```python
from build123d import *

# Parameters (mm, degrees)
F0_W     = 15
F0_H     = 22.5
F1_DEPTH = 0.75
F2_DEPTH = 2


with BuildPart() as f1:
    # F0 (on Top) → F1 (new body)
    with BuildSketch(Plane.XY):
        with Locations((-24.588022, -15.75)):
            Rectangle(F0_W, F0_H)
        Polygon((-18.888022, -25), (-30.888022, -25), (-30.888022, -10), (-21.388022, -10), (-18.888022, -12.5), align=None, mode=Mode.SUBTRACT)
    extrude(amount=F1_DEPTH)

    # F0 (on Top) → F2 (join)
    with BuildSketch(Plane.XY):
        Polygon((-32.088022, 3), (-32.088022, -4.5), (-17.088022, -4.5), (-17.088022, 0), (-20.088022, 3), align=None)
    extrude(amount=F2_DEPTH)


solid = f1.part
```
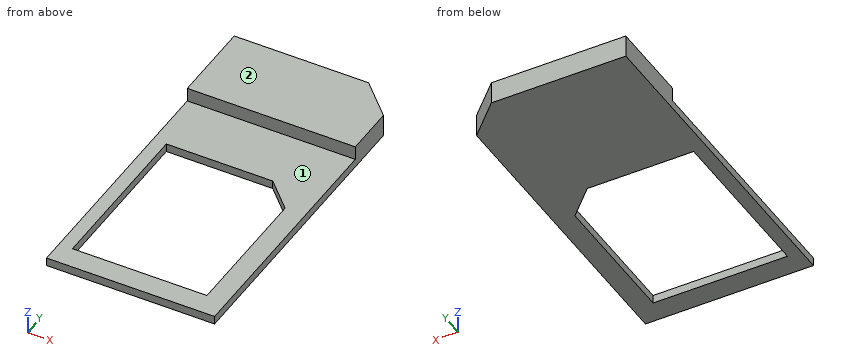
The listing builds one solid part. Answer for the finished solid, in the listing's coordinates (mm). Face numbers are marked on the shaded views. A direction names the side the tool comes from. Give positions to 0.01 mm unless a question says otherwise; leave off trailing zeros. Order: outer loops, then holes, each group sorted by start corner. A loop starts at its lowest first (then second) coordinate and runs counter-clockwise, first axis right, second up.
Item 1: Given pin 1 Ø1 at (x, z) = (-23.5, 1) entering from -Y; pin 2 Ø4.5 at (x, y) = (-22.5, -18.5) entering from +Z, each flat-ended and moving along its own axis, determine where each tip first touches the part or whether it passes through.
From the geometry:
pin 1: stops at y = -27
pin 2: passes through
Item 2: The part is cut by section B-B, the plane z = 0.45. Give the vertices of the cut face in (x, y).
From the geometry:
outline: (-32.09, -27) - (-17.09, -27) - (-17.09, 0) - (-20.09, 3) - (-32.09, 3) - close; hole (-30.89, -25) - (-18.89, -25) - (-18.89, -12.5) - (-21.39, -10) - (-30.89, -10) - close
Item 3: The part is cut by section C-C, the plane x = -29.5. Give the vertices of the cut face in (y, z), and give its area (3 significant figures).
From the geometry:
outline: (-27, 0) - (-25, 0) - (-25, 0.75) - (-27, 0.75) - close; (-10, 0) - (3, 0) - (3, 2) - (-4.5, 2) - (-4.5, 0.75) - (-10, 0.75) - close
area: 20.6 mm2
Item 4: Which of the six approach directions +Z, -Z, +X, -X, +Y, -Y give full straight-line access (tool end or side, diameter ignored) to the marked faces 1 and 2?
From the geometry:
face 1: +Z, +X, -X, -Y
face 2: +Z, +X, -X, +Y, -Y
Item 5: Find the intervals of material crossed by probe 1 along Y at (x, z) = (-25.5, 0.35); probe 2 along Y at (x, z) = (-22.25, 1.35); probe 3 along Z at (x, y) = (-31.25, -15), in increasing order.
From the geometry:
probe 1: y = -27 to -25, -10 to 3
probe 2: y = -4.5 to 3
probe 3: z = 0 to 0.75
Item 6: The part is cut by section D-D, the plane y = -11. Give the vertices of the cut face in (x, z), and give its area (4 significant figures).
From the geometry:
outline: (-32.09, 0) - (-30.89, 0) - (-30.89, 0.75) - (-32.09, 0.75) - close; (-20.39, 0) - (-17.09, 0) - (-17.09, 0.75) - (-20.39, 0.75) - close
area: 3.375 mm2
Item 7: The part is cut by section A-A, the plane y = -15.75. Give the vertices of the cut face in (x, z), and give its area (3 significant figures).
From the geometry:
outline: (-32.09, 0) - (-30.89, 0) - (-30.89, 0.75) - (-32.09, 0.75) - close; (-18.89, 0) - (-17.09, 0) - (-17.09, 0.75) - (-18.89, 0.75) - close
area: 2.25 mm2
